from build123d import *

# Parameters (mm, degrees)
BOSS_EXTRUDE1_DEPTH = 21
SKETCH2_R           = 44.092659675
SKETCH2_R_2         = 35.039506693
BOSS_EXTRUDE2_DEPTH = 14.465745569
BOSS_EXTRUDE3_START = -14.465745569
SKETCH4_R           = 44.092659675
SKETCH4_R_2         = 35.039506693
BOSS_EXTRUDE3_DEPTH = 14.465745569


with BuildPart() as part:
    # Sketch1 → Boss-Extrude1 (new body)
    with BuildSketch(Plane(origin=(0, 0, 0), x_dir=(1, 0, 0), z_dir=(0, 1, 0))):
        with BuildLine():
            Line((0, 37.924000209), (23.712323124, 37.924000209))
            Line((23.712323124, 37.924000209), (23.712323124, 23.45825464))
            Line((23.712323124, 23.45825464), (0, 23.45825464))
            ThreePointArc((0, 23.45825464), (-23.45825464, 0), (0, -23.45825464))
            Line((0, -23.45825464), (23.712323124, -23.45825464))
            Line((23.712323124, -23.45825464), (23.712323124, -37.924000209))
            Line((23.712323124, -37.924000209), (0, -37.924000209))
            ThreePointArc((0, -37.924000209), (-16.561988679, -34.116423067), (-29.798323461, -23.45825464))
            Line((-29.798323461, -23.45825464), (-29.798323461, -23.712323124))
            Line((-29.798323461, -23.712323124), (-156.054398777, -23.712323124))
            Line((-156.054398777, -23.712323124), (-156.054398777, 23.45825464))
            Line((-156.054398777, 23.45825464), (-29.798323461, 23.45825464))
            ThreePointArc((-29.798323461, 23.45825464), (-16.561988679, 34.116423067), (0, 37.924000209))
        make_face()
    extrude(amount=BOSS_EXTRUDE1_DEPTH)

    # Sketch2 → Boss-Extrude2 (add)
    with BuildSketch(Plane.XY.offset(-23.45825464)):
        with Locations((66.225280873, 10.5)):
            Circle(SKETCH2_R)
        with Locations((66.225280873, 10.5)):
            Circle(SKETCH2_R_2, mode=Mode.SUBTRACT)
    extrude(amount=-BOSS_EXTRUDE2_DEPTH)

    # Sketch4 → Boss-Extrude3 (add)
    with BuildSketch(Plane(origin=(0, 0, 23.45825464), x_dir=(-1, 0, 0), z_dir=(0, 0, -1)).offset(BOSS_EXTRUDE3_START)):
        with Locations((-66.225280873, 10.5)):
            Circle(SKETCH4_R)
        with Locations(Location((-66.225280873, 10.5, 0), (0, 0, 180))):
            Circle(SKETCH4_R_2, mode=Mode.SUBTRACT)
    extrude(amount=BOSS_EXTRUDE3_DEPTH)


solid = part.part
For this review, take the finished solid that the model builds, in its own axes (mm). A direction names the side the tool comes from. Give positions to 0.01 mm unless a question says otherwise; leave off trailing zeros. Order: outer loops, then holes, each group sorted by start corner. A loop starts at its lowest first (then second) coordinate and runs counter-clockwise, first axis right, second up. Notation, with made-up numbers: (-28.5, -16.75) -> (-3.5, -16.75) arc R14 cw to (-3.5, 2.25) -> close; hole circle Ø7 at (82.5, 1.25). An arc over 180 degrees is marked (long way). Write item = value, one per line.
1) Draft analysis for pull direction Y (two halves, no side actions). For faces 1 (the face through (-65, 0, -1)), 2 (the face through (99.65, -0.02, 30.79)), 3 (the face through (-92, 10, 23.712)), state which applies: pulls with the +Y half, pulls with the -Y half, needs draft (parallel to the pull), parting line crosses it, or undercut.
Findings:
face_1 = pulls with the -Y half
face_2 = undercut
face_3 = needs draft
2) For faces 4 (the face through (30, 14, -23.458)), 5 (the face through (-156.054, 10, 0)), 6 (the face through (-65, 21, -1)), 7 (the face through (-94, 10, -23.458)), 8 (the face through (30, 14, -37.924)), list the 3-axis set-ups (+Z, -Z, +X, -X, +Y, -Y) from which the entire face can be reached by the end or side of a thin tool; tool diameter is ignored.
Findings:
face_4 = +X, +Y, -Y
face_5 = +Z, -Z, -X, +Y, -Y
face_6 = +Z, -Z, -X, +Y
face_7 = -Z, -X, +Y, -Y
face_8 = -Z, +X, -X, +Y, -Y
3) We need section D-D, the plane z = 0. Give the boundary of the cut face in (x, y), and give its area (3 significant figures).
Findings:
outline = (-156.05, 0) -> (-23.46, 0) -> (-23.46, 21) -> (-156.05, 21) -> close
area = 2,780 mm^2
4) We need section A-A, the plane y = 35. Give the boundary of the cut face in (x, z) (3 decimals), and give its area (3 significant figures).
Findings:
outline = (29.566, -37.924) -> (41.175, -37.924) -> (41.175, -23.458) -> (29.566, -23.458) -> close; (29.566, 23.458) -> (41.175, 23.458) -> (41.175, 37.924) -> (29.566, 37.924) -> close; (91.276, -37.924) -> (102.885, -37.924) -> (102.885, -23.458) -> (91.276, -23.458) -> close; (91.276, 23.458) -> (102.885, 23.458) -> (102.885, 37.924) -> (91.276, 37.924) -> close
area = 672 mm^2
5) We need section B-B, the plane x = 60. Give the boundary of the cut face in (y, z), and give its area (3 significant figures).
Findings:
outline = (-33.15, -37.92) -> (-23.98, -37.92) -> (-23.98, -23.46) -> (-33.15, -23.46) -> close; (-33.15, 23.46) -> (-23.98, 23.46) -> (-23.98, 37.92) -> (-33.15, 37.92) -> close; (44.98, -37.92) -> (54.15, -37.92) -> (54.15, -23.46) -> (44.98, -23.46) -> close; (44.98, 23.46) -> (54.15, 23.46) -> (54.15, 37.92) -> (44.98, 37.92) -> close
area = 531 mm^2
6) We need section C-C, the plane y = 10.5. Give the boundary of the cut face in (x, z), and give its area (3 significant figures).
Findings:
outline = (-156.05, -23.46) -> (-29.8, -23.46) arc R37.92 ccw to (0, -37.92) -> (31.19, -37.92) -> (31.19, -23.46) -> (0, -23.46) arc R23.46 cw to (0, 23.46) -> (31.19, 23.46) -> (31.19, 37.92) -> (0, 37.92) arc R37.92 ccw to (-29.8, 23.46) -> (-29.8, 23.71) -> (-156.05, 23.71) -> close; (101.26, -37.92) -> (110.32, -37.92) -> (110.32, -23.46) -> (101.26, -23.46) -> close; (101.26, 23.46) -> (110.32, 23.46) -> (110.32, 37.92) -> (101.26, 37.92) -> close
area = 8,250 mm^2
7) To check wall thickness, follow L1, parallel to Z at x = 31.5, y = 30; L2, parallel to X at y = 10, z = -29; L3, parallel to Y at x = -107, z = -19. State the ranges of each line that lie inside material, in increasing order. Write a range as from..to.
Findings:
L1 = -37.92..-23.46, 23.46..37.92
L2 = -24.44..31.19, 101.26..110.32
L3 = 0..21
8) Insertion check: pin 1 (2 mm diameter, centred on y = 35.5, z = 28.5, fed in from -X); pin 2 (10.5 mm diameter, centred on x = -99.5, y = 10.5, fed in from -Z); pin 3 (6.5 mm diameter, centred on x = -69, y = 10, fed in from +Z). Each pin has a flat end and moves straight along its axis. Give the tip position at first contact, or say it passes through.
Findings:
pin_1 = 29.24
pin_2 = -23.46
pin_3 = 23.71
